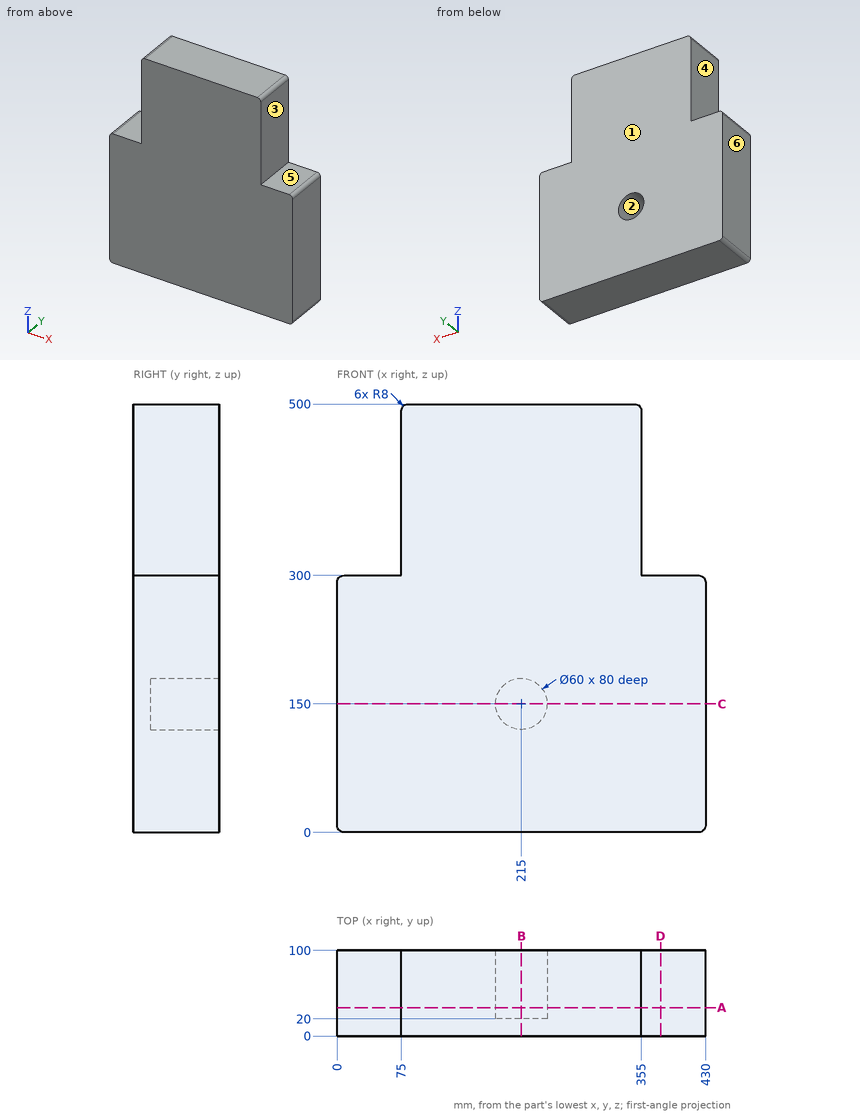
Print and shaded views of the part. All mm, measured from the part's lowest x, y and z. A direction names the side the tool comes from. Give positions to 0.01 mm unless a question says otherwise; leave off trailing zeros. Write each loop counter-clockwise with the first axis right and the second up, starting at its lowest first coordinate (ties: lowest second). Pieces come first, ordered by that corner, then holes. Notation, with made-up numbers: (74.25, 44.25) -> (110.25, 44.25) arc R8 cw to (110.25, 56.25) -> close; hole circle Ø8 at (5.5, -37). An arc over 180 degrees is marked (long way). Use CSV: the item, a comma, the result in double quotes. Start each with the question number.
1) Tool access for the marked faces 4, 5 and 6: list every direction of +Z, -Z, +X, -X, +Y, -Y with a clear straight run to the whole face (end or side of a thin tool).
2) Drill centre lines: L1, parallel to X at y = 43, z = 150; L2, parallel to X at y = 5.5, z = 374; L3, parallel to Z at x = 215, y = 44. Where is each one in solid material? Low to high.
3) Pin check, flat tip, straight feed: P1, Ø20, axis at x = 40, y = 51.5, coming from the +Z side. Stop position of the tip, or through.
4) Cut at C-C on z = 150. List the corners of the cut face in (x, y), plus the area to 3 significant figures.
5) Two-plate mould, pull along X, no slides. Class the marked faces 1, 2 and 3: released by +X, released by -X, zero draft, split by the parting line, or undercut.
6) Cut at B-B on x = 215. List the corners of the cut face in (y, z), plus the area to 3 significant figures.
7) Cut at D-D on x = 377.5. List the corners of the cut face in (y, z), plus the area to 3 significant figures.
8) Cut at A-A on y = 33. List the corners of the cut face in (x, z).
Final values:
1,face 4,"+Z, -X, +Y, -Y"
1,face 5,"+Z, +X, +Y, -Y"
1,face 6,"+Z, -Z, -X, +Y, -Y"
2,L1,"x = 0 to 185, 245 to 430"
2,L2,"x = 75 to 355"
2,L3,"z = 0 to 120, 180 to 500"
3,P1,"stops at z = 300"
4,outline,"(0, 0) -> (430, 0) -> (430, 100) -> (245, 100) -> (245, 20) -> (185, 20) -> (185, 100) -> (0, 100) -> close"
4,area,"38,200 mm2"
5,face 1,"zero draft"
5,face 2,"undercut"
5,face 3,"released by +X"
6,outline,"(0, 0) -> (100, 0) -> (100, 120) -> (20, 120) -> (20, 180) -> (100, 180) -> (100, 500) -> (0, 500) -> close"
6,area,"45,200 mm2"
7,outline,"(0, 0) -> (100, 0) -> (100, 300) -> (0, 300) -> close"
7,area,"30,000 mm2"
8,outline,"(0, 8) arc R8 ccw to (8, 0) -> (422, 0) arc R8 ccw to (430, 8) -> (430, 292) arc R8 ccw to (422, 300) -> (355, 300) -> (355, 492) arc R8 ccw to (347, 500) -> (83, 500) arc R8 ccw to (75, 492) -> (75, 300) -> (8, 300) arc R8 ccw to (0, 292) -> close; hole circle Ø60 at (215, 150)"
